from build123d import *

# Parameters (mm, degrees)
CYLINDER048_R             = 31
CYLINDER048_DEPTH         = 6
CYLINDER047_R             = 34
CYLINDER047_DEPTH         = 3
FUSION025_PLACEMENT_ANGLE = 180


with BuildPart() as cylinder048:
    # Cylinder048 → Cylinder048 (new body)
    with BuildSketch(Plane.XY):
        Circle(CYLINDER048_R)
    extrude(amount=CYLINDER048_DEPTH)


with BuildPart() as cap:
    # Cylinder047 → Cylinder047 (new body)
    with BuildSketch(Plane.XY):
        Circle(CYLINDER047_R)
    extrude(amount=CYLINDER047_DEPTH)

    # Fusion025: union Cylinder048
    add(cylinder048.part)


with BuildPart() as cap_1:
    # Fusion025 placement: moved
    add(cap.part.moved(Location((39, 41, 88))).rotate(Axis((39, 41, 88), (1, 0, 0)), FUSION025_PLACEMENT_ANGLE))


solid = cap_1.part
Could you check a few things on this model? Use its own coordinates, in mm. A direction names the side the tool comes from. Round coordinates to 2 decimals unless told otherwise and drop trailing zeros. Order: outer loops, then holes, each group sorted by start corner. A loop starts at its lowest first (then second) coordinate and runs counter-clockwise, first axis right, second up.
Q1. Imagine slicing it at A-A, the plane y = 41. List the corners of the cut face in (x, z) for me.
Geometry says:
outline: (5, 85) - (8, 85) - (8, 82) - (70, 82) - (70, 85) - (73, 85) - (73, 88) - (5, 88) - close
Q2. Imagine slicing it at C-C, the plane z = 84.1. List the corners of the cut face in (x, y) for me.
Geometry says:
outline: circle Ø62 at (39, 41)
Q3. Imagine slicing it at B-B, the plane x = 39. List the corners of the cut face in (y, z) for me, then the cut area to 3 significant figures.
Geometry says:
outline: (7, 85) - (10, 85) - (10, 82) - (72, 82) - (72, 85) - (75, 85) - (75, 88) - (7, 88) - close
area: 390 mm2
Q4. Please list where these lines run through material, in increasing order: probe 1 along X at (y, z) = (40, 85.8); probe 2 along X at (y, z) = (72, 86.2); probe 3 along Z at (x, y) = (9, 49.5).
Geometry says:
probe 1: x = 5.01 to 72.99
probe 2: x = 25.04 to 52.96
probe 3: z = 85 to 88
Q5. I'm going to push flat-ended pins straight in: P1, Ø1, axis at x = 30.5, z = 84, coming from the -Y side; P2, Ø1, axis at x = 57, z = 86.5, coming from the +Y side. Where does each tip first touch, or does it pass through?
Geometry says:
P1: stops at y = 11.05
P2: stops at y = 70.15
Q6. Which directions (+Z, -Z, +X, -X, +Y, -Y) give clear straight access to the entire face, cutting with the end or side of a thin tool? Please do faces 1 (the face through (39, 41, 88)), 2 (the face through (67, 56, 85)).
Geometry says:
face 1: +Z, +X, -X, +Y, -Y
face 2: -Z
